Study the drawing (mm; zero at the part's minimum x, y, z) and answer. Give positions to 0.01 mm unless a question says otherwise; leave off trailing zeros. Write each loop counter-clockwise with the first axis right and the second up, starting at its lowest first coordinate (ties: lowest second). Pieces come first, ordered by that corner, then holes.
1) Find section D-D (z = 69). Determine the outline of the cut face in (x, y), plus the area to 3 significant figures.
2) Find section C-C (z = 25). Determine the outline of the cut face in (x, y).
3) Straight lines are drawn through the part: probe 1 along Y at (x, z) = (63.5, 119); probe 2 along X at (y, z) = (63, 73) (1 decimal); probe 3 along Y at (x, z) = (63.5, 37). For each, find the intervals that lie inside material, in ascending order.
4) Find section A-A (x = 63.5). Determine the outline of the cut face in (y, z).
5) Determine the mould class of the marked faces 1, 2 and 3 for opening direction Y: pulls with the +Y half, pulls with the -Y half, needs draft (parallel to the pull), parting line crosses it, or undercut.
6) Given pin 1 Ø12 at (x, z) = (73, 78) entering from -Y; pin 2 Ø12 at (x, z) = (86, 137) entering from -Y; pin 3 Ø10 at (y, z) = (33, 69.5) entering from -X, each flat-ended and moving along its own axis, determine where each tip first touches the part or whether it passes through.
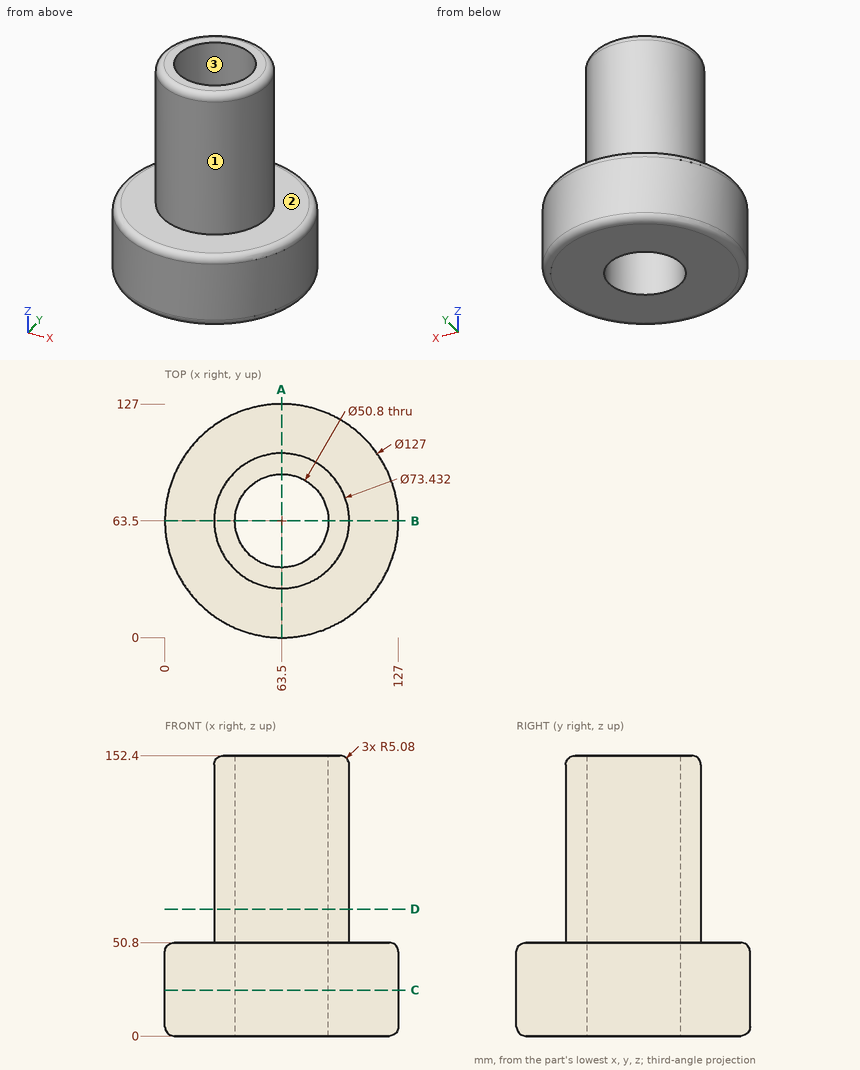
Results:
1. outline: circle Ø73.43 at (63.5, 63.5); hole circle Ø50.8 at (63.5, 63.5)
1. area: 2,210 mm2
2. outline: circle Ø127 at (63.5, 63.5); hole circle Ø50.8 at (63.5, 63.5)
3. probe 1: y = 26.78 to 38.1, 88.9 to 100.22
3. probe 2: x = 26.8 to 38.1, 88.9 to 100.2
3. probe 3: y = 0 to 38.1, 88.9 to 127
4. outline: (0, 5.08) arc R5.08 ccw to (5.08, 0) - (38.1, 0) - (38.1, 152.4) - (31.86, 152.4) arc R5.08 ccw to (26.78, 147.32) - (26.78, 50.8) - (5.08, 50.8) arc R5.08 ccw to (0, 45.72) - close; (88.9, 0) - (121.92, 0) arc R5.08 ccw to (127, 5.08) - (127, 45.72) arc R5.08 ccw to (121.92, 50.8) - (100.22, 50.8) - (100.22, 147.32) arc R5.08 ccw to (95.14, 152.4) - (88.9, 152.4) - close
5. face 1: parting line crosses it
5. face 2: needs draft
5. face 3: undercut
6. pin 1: stops at y = 26.95
6. pin 2: stops at y = 30.7
6. pin 3: stops at x = 37.08
